The listing builds one solid part. Answer for the finished solid, in the listing's coordinates (mm). Face numbers are marked on the shaded views. Coordinates: 2 decimals unless noted, no trailing zeros. Loops run counter-clockwise (first coordinate to the right, second up) from the corner with the lowest first, then second, coordinate; pieces in that order, holes last. Notation, with made-up numbers: M -27.5,-15.75 L 21.5,-15.75 A12 ccw 21.5,1.25 Z; hole C -5.75,83.25 d7. An arc over 180 degrees is marked long. Answer as a JSON object with one key per item and string values. Group by question number.
1. A cutting plane is placed at B-B on z = 1.3. Give the vertices of the cut face in (x, y).
2. A cutting plane is placed at D-D on z = 2.15. Give the vertices of the cut face in (x, y), and give its area (3 significant figures).
3. Determine the mould class of the marked faces 1, 2 and 3 for opening direction X: released by +X, released by -X, zero draft, split by the parting line, or undercut.
4. A cutting plane is placed at C-C on y = -2. Give the vertices of the cut face in (x, z), and give its area (3 significant figures).
5. Straight lines are drawn through the part: L1, parallel to Y at x = -0.5, z = 2.55; L2, parallel to Y at x = 0.25, z = 2.4; L3, parallel to X at y = -2, z = 2.85. For each, find the intervals that lie inside material, in ascending order.
6. A cutting plane is placed at A-A on y = 0. Give the vertices of the cut face in (x, z).
7. Given pin 1 (1.5 mm diameter, centred on y = 1, z = 2.5, fed in from +X), flat-ended and moving along its own axis, determine where the tip first touches the part or whether it passes through.
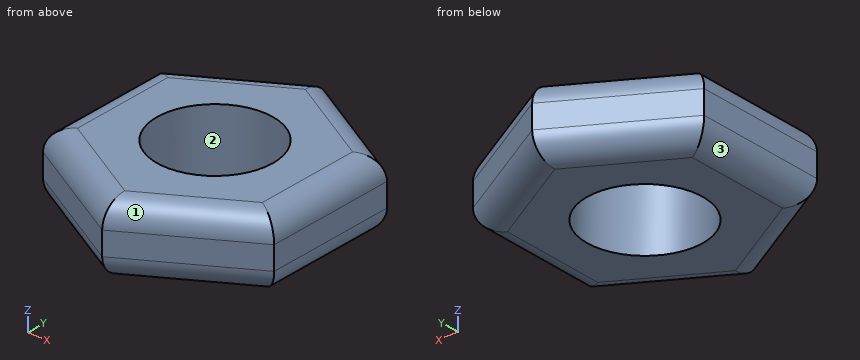
from build123d import *

# Parameters (mm, degrees)
F0_R     = 2.5
F1_DEPTH = 3
F2_R     = 1


with BuildPart() as f1:
    # F0 (on Top) → F1 (new body)
    with BuildSketch(Plane.XY):
        Polygon((-5, 2.886751), (-5, -2.886751), (0, -5.773503), (5, -2.886751), (5, 2.886751), (0, 5.773503), align=None)
        Circle(F0_R, mode=Mode.SUBTRACT)
    extrude(amount=F1_DEPTH)

    # F2
    f2_edges = [f1.edges().sort_by_distance(p)[0] for p in [
        (5, 0, 0),
        (2.5, 4.330127, 0),
        (-2.5, 4.330127, 0),
        (-5, 0, 0),
        (-2.5, -4.330127, 0),
        (2.5, -4.330127, 0),
        (5, 0, 3),
        (2.5, -4.330127, 3),
        (-2.5, -4.330127, 3),
        (-5, 0, 3),
        (-2.5, 4.330127, 3),
        (2.5, 4.330127, 3),
    ]]
    fillet(f2_edges, radius=F2_R)


solid = f1.part
From the geometry:
{
 "1": {"outline": "M -5,-2.89 L 0,-5.77 L 5,-2.89 L 5,2.89 L 0,5.77 L -5,2.89 Z; hole C 0,0 d5"},
 "2": {"outline": "M -4.99,-2.88 L 0,-5.76 L 4.99,-2.88 L 4.99,2.88 L 0,5.76 L -4.99,2.88 Z; hole C 0,0 d5", "area": "66.6 mm²"},
 "3": {"face 1": "released by +X", "face 2": "undercut", "face 3": "released by -X"},
 "4": {"outline": "M -5,1 A1 ccw -4,0 L -1.5,0 L -1.5,3 L -4,3 A1 ccw -5,2 Z; M 1.5,0 L 4,0 A1 ccw 5,1 L 5,2 A1 ccw 4,3 L 1.5,3 Z", "area": "20.1 mm²"},
 "5": {"L1": "y = -5.29 to -2.45, 2.45 to 5.29", "L2": "y = -5.53 to -2.49, 2.49 to 5.53", "L3": "x = -4.53 to -1.5, 1.5 to 4.53"},
 "6": {"outline": "M -5,1 A1 ccw -4,0 L -2.5,0 L -2.5,3 L -4,3 A1 ccw -5,2 Z; M 2.5,0 L 4,0 A1 ccw 5,1 L 5,2 A1 ccw 4,3 L 2.5,3 Z"},
 "7": {"pin 1": "stops at x = 5"}
}
